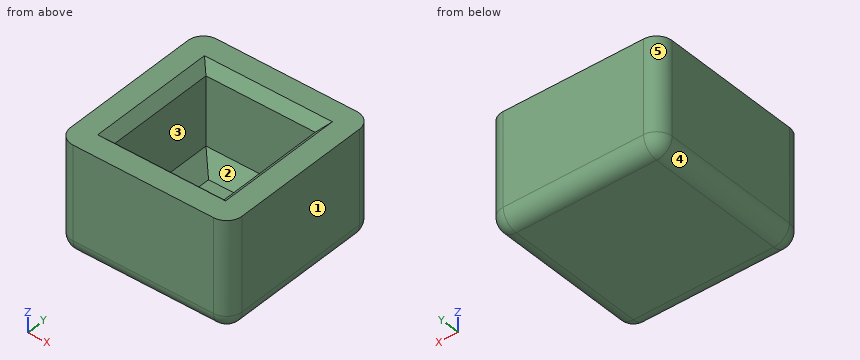
from build123d import *

# Parameters (mm, degrees)
F0_W     = 55
F0_H     = 55
F0_W_2   = 35
F0_H_2   = 35
F1_DEPTH = 5
F2_DEPTH = 30
F3_R     = 5
F4_SIZE  = 3
F5_SIZE  = 5


with BuildPart() as f1:
    # F0 (on Top) → F1 (new body)
    with BuildSketch(Plane.XY):
        Rectangle(F0_W, F0_H)
        Rectangle(F0_W_2, F0_H_2, mode=Mode.SUBTRACT)
        Rectangle(F0_W_2, F0_H_2)
    extrude(amount=-F1_DEPTH)

    # F0 (on Top) → F2 (join)
    with BuildSketch(Plane.XY):
        Rectangle(F0_W, F0_H)
        Rectangle(F0_W_2, F0_H_2, mode=Mode.SUBTRACT)
    extrude(amount=F2_DEPTH)

    # F3
    f3_edges = [f1.edges().sort_by_distance(p)[0] for p in [
        (0, -27.5, -5),
        (27.5, 0, -5),
        (0, 27.5, -5),
        (-27.5, 0, -5),
        (27.5, 27.5, 12.5),
        (-27.5, 27.5, 12.5),
        (-27.5, -27.5, 12.5),
        (27.5, -27.5, 12.5),
    ]]
    fillet(f3_edges, radius=F3_R)

    # F4
    f4_edges = [f1.edges().sort_by_distance(p)[0] for p in [
        (-17.5, 0, 30),
        (0, -17.5, 30),
        (17.5, 0, 30),
        (0, 17.5, 30),
    ]]
    chamfer(f4_edges, length=F4_SIZE)

    # F5
    f5_edges = [f1.edges().sort_by_distance(p)[0] for p in [
        (17.5, 0, 0),
        (0, -17.5, 0),
        (-17.5, 0, 0),
        (0, 17.5, 0),
    ]]
    chamfer(f5_edges, length=F5_SIZE)


solid = f1.part
Verification items for the finished model (mm, model axes). Face numbers are marked on the shaded views. A direction names the side the tool comes from. Give positions to 0.01 mm unless a question says otherwise; leave off trailing zeros. Write each loop counter-clockwise with the first axis right and the second up, starting at its lowest first coordinate (ties: lowest second). Pieces come first, ordered by that corner, then holes. Notation, with made-up numbers: M -22,31.5 L -1,31.5 A24 ccw -1,49.5 Z; hole C 75.25,20.5 d10. An arc over 180 degrees is marked long. Put each result on its own line as item: value. Start each with the question number.
1. Scan lines: line 1 along X through (y, z) = (10, 26); line 2 along Z through (x, y) = (18, 16.5). Record each from-to range of solid material in increasing order. Write a range as [from, to].
2. Draft check along Y on the marked faces 3, 4 and 5. Enter one of: +Y half, -Y half, draft (parallel to the pull), parting line (faces both ways), or undercut.
3. Section check D-D (z = 28). Record the cut outline in (x, y).
4. Section check A-A (z = 3). Record the cut outline in (x, y).
5. Section check B-B (y = -1.5). Record the cut outline in (x, z), and give its area (3 significant figures).
6. Set-up check for the marked faces 1 and 2: record each of +Z, -Z, +X, -X, +Y, -Y from which the full face is reachable in a straight line by a thin tool's end or side.
7. Go/stop test with flat-tipped pins: pin 1 Ø7.5 at (x, y) = (2.5, 5) entering from +Z; pin 2 Ø1.5 at (x, y) = (17.5, 4.5) entering from +Z. Record where each tip stops, or that it passes through.
Answer list:
1. line 1: [-27.5, -17.5], [17.5, 27.5]
1. line 2: [-5, 27.5]
2. face 3: undercut
2. face 4: draft
2. face 5: +Y half
3. outline: M -27.5,-22.5 A5 ccw -22.5,-27.5 L 22.5,-27.5 A5 ccw 27.5,-22.5 L 27.5,22.5 A5 ccw 22.5,27.5 L -22.5,27.5 A5 ccw -27.5,22.5 Z; hole M -18.5,-18.5 L 18.5,-18.5 L 18.5,18.5 L -18.5,18.5 Z
4. outline: M -27.5,-22.5 A5 ccw -22.5,-27.5 L 22.5,-27.5 A5 ccw 27.5,-22.5 L 27.5,22.5 A5 ccw 22.5,27.5 L -22.5,27.5 A5 ccw -27.5,22.5 Z; hole M -15.5,-15.5 L 15.5,-15.5 L 15.5,15.5 L -15.5,15.5 Z
5. outline: M -27.5,0 A5 ccw -22.5,-5 L 22.5,-5 A5 ccw 27.5,0 L 27.5,30 L 20.5,30 L 17.5,27 L 17.5,5 L 12.5,0 L -12.5,0 L -17.5,5 L -17.5,27 L -20.5,30 L -27.5,30 Z
5. area: 880 mm2
6. face 1: +Z, -Z, +X, +Y, -Y
6. face 2: +Z
7. pin 1: z = 0
7. pin 2: z = 27.75
